Verification items for the finished model (mm, model axes). A direction names the side the tool comes from. Give positions to 0.01 mm unless a question says otherwise; leave off trailing zeros. Order: outer loops, then holes, each group sorted by start corner. A loop starts at its lowest first (then second) coordinate and runs counter-clockwise, first axis right, second up. Notation, with made-up numbers: (-6, 43) - (45, 43) arc R21 cw to (45, 58) - close; hole circle Ø6 at (35.5, -7). An arc over 180 degrees is marked (long way). Answer as a JSON object with one key per item and string values.
```python
from build123d import *

# Parameters (mm, degrees)
SKETCH_2_W      = 12
SKETCH_2_H      = 12
EXTRUDE_1_DEPTH = 9
CHAMFER_1_SIZE  = 1
FILLET_1_R      = 1
FILLET_2_R      = 0.5
CHAMFER_2_SIZE  = 2


with BuildPart() as part:
    # Эскиз1 → Повернуть1 (revolve)
    with BuildSketch(Plane.XY, mode=Mode.PRIVATE) as revolve_1_sk:
        with BuildLine():
            Line((0, 6), (0, 6.535898385))
            Line((0, 6.535898385), (6, 10))
            Line((6, 10), (33, 10))
            Line((33, 10), (33, 6))
            Line((33, 6), (42, 6))
            Line((42, 6), (42, 4.75))
            Line((42, 4.75), (46, 4.75))
            Line((46, 4.75), (47.25, 6))
            Line((47.25, 6), (60, 6))
            Line((60, 6), (60, 0))
            Line((60, 0), (6, 0))
            ThreePointArc((6, 0), (4.242640687, 4.242640687), (0, 6))
        make_face()
    revolve(revolve_1_sk.sketch.rotate(Axis((0, 0, 0), (1, 0, 0)), 180), axis=Axis((0, 0, 0), (1, 0, 0)))

    # Эскиз2 → Бобышка-Вытянуть1 (add)
    with BuildSketch(Plane(origin=(33, 0, 0), x_dir=(0, 0, -1), z_dir=(1, 0, 0))):
        Rectangle(SKETCH_2_W, SKETCH_2_H)
    extrude(amount=EXTRUDE_1_DEPTH)

    # Фаска1
    chamfer_1_edges = [part.edges().sort_by_distance(p)[0] for p in [
        (37.5, -6, 6),
        (37.5, 6, 6),
        (37.5, 6, -6),
        (37.5, -6, -6),
    ]]
    chamfer(chamfer_1_edges, length=CHAMFER_1_SIZE)

    # Скругление1
    fillet_1_edges = [part.edges().sort_by_distance(p)[0] for p in [
        (42, 4.75, 0),
    ]]
    fillet(fillet_1_edges, radius=FILLET_1_R)

    # Скругление2
    fillet_2_edges = [part.edges().sort_by_distance(p)[0] for p in [
        (46, 4.75, 0),
    ]]
    fillet(fillet_2_edges, radius=FILLET_2_R)

    # Фаска2
    chamfer_2_edges = [part.edges().sort_by_distance(p)[0] for p in [
        (60, 6, 0),
    ]]
    chamfer(chamfer_2_edges, length=CHAMFER_2_SIZE)


solid = part.part
```
(1) Gauge pin test, flat ends, axial feed: pin 1 Ø7 at (x, z) = (37.5, 2) entering from +Y; pin 2 Ø4 at (x, y) = (50, 4.5) entering from +Z; pin 3 Ø2.5 at (x, y) = (36, 1.5) entering from +Z. Record the tip position at first contact, or that the pin passes through.
Computed values:
{"pin 1": "stops at y = 6", "pin 2": "stops at z = 5.45", "pin 3": "stops at z = 6"}
(2) Material ranges on line 1 along Y through (x, z) = (24, 8); line 2 along Y through (x, z) = (4.5, 1.5); line 3 along X through (y, z) = (5.25, 1), recorded low to high. Write a range as [from, to].
Computed values:
{"line 1": "y = [-6, 6]", "line 2": "y = [-9.01, -3.67], [3.67, 9.01]", "line 3": "x = [2.73, 42.09], [46.59, 58.66]"}
(3) Access from +Z, -Z, +X, -X, +Y, -Y to the whole of each face (thin tool, end or side, straight path). Record for faces 4 (the flat face through (33, -7, 0)), 5 (the flat face through (37.4, -5.5, -5.5)), 6 (the flat face through (37, 0, -6)), 7 (the flat face through (42, 5.8, 1.4)).
Computed values:
{"face 4": "+X", "face 5": "-Z, +X, -Y", "face 6": "-Z, +X, +Y, -Y", "face 7": "none"}
(4) Release check for a two-part mould opening along X. For faces 1 (the cylindrical face through (44.416, 1.03, 4.637)), 2 (the conical face through (0.4, 1.5, 6.6)), 3 (the cylindrical face through (20, 10, 0)) record: pulls with the +X half, pulls with the -X half, needs draft (parallel to the pull), parting line crosses it, or undercut.
Computed values:
{"face 1": "undercut", "face 2": "pulls with the -X half", "face 3": "needs draft"}
(5) Section check A-A (x = 8). Record the cut outline in (y, z), then the cut area to 3 significant figures.
Computed values:
{"outline": "circle Ø20 at (0, 0)", "area": "314 mm²"}
